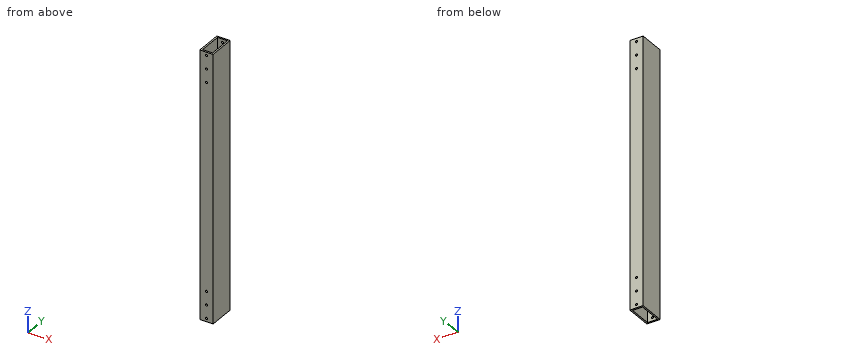
Autodesk Inventor part; units mm, degrees
ref_plane "Start Plane" through (0, 0, 0) normal (0, 0, 1) x (1, 0, 0)
ref_plane "End Plane" through (0, 0, 508) normal (0, 0, 1) x (1, 0, 0)
ref_plane "YZ Plane" through (0, 0, 0) normal (1, 0, 0) x (0, 1, 0)
ref_plane "Start Plane" through (0, 0, 0) normal (0, 0, 1) x (1, 0, 0)
ref_plane "End Plane" through (0, 0, 508) normal (0, 0, 1) x (1, 0, 0)
sketch "Sketch" plane through (0, 0, 0) normal (0, 0, 1) x (1, 0, 0)
  line L0 (-12.7, -25.4) -> (12.7, -25.4)
  line L1 (12.7, -25.4) -> (12.7, 25.4)
  line L2 (12.7, 25.4) -> (-12.7, 25.4)
  line L3 (-12.7, 25.4) -> (-12.7, -25.4)
  line L4 (-12.7, -25.4) -> (12.7, 25.4) construction
  line L5 (12.7, -25.4) -> (-12.7, 25.4) construction
  line L6 (-9.525, -22.225) -> (9.525, -22.225)
  line L7 (9.525, -22.225) -> (9.525, 22.225)
  line L8 (9.525, 22.225) -> (-9.525, 22.225)
  line L9 (-9.525, 22.225) -> (-9.525, -22.225)
  line L10 (-9.525, -22.225) -> (9.525, 22.225) construction
  line L11 (9.525, -22.225) -> (-9.525, 22.225) construction
  point P0 (0, 0)
  dimension "d0" = 25.4
  dimension "d1" = 50.8
  dimension "d2" = 3.175
  dimension "d3" = 3.175
extrude "Body" add sketch "Sketch" along normal up to surface (508 mm away) from surface at 0
sketch "Sketch6" plane through (0, 0, 0) normal (0, 0, 1) x (1, 0, 0)
  line L0 (0, 0) -> (10, 0)
ref_plane "Work Plane5" through (0, 0, 0) normal (0, -1, 0) x (1, 0, 0)
sketch "Sketch7" plane through (0, 0, 0) normal (0, -1, 0) x (1, 0, 0)
  line L0 (-2, 0) -> (12, 0)
  line L1 (-2, 508) -> (12, 508)
  dimension "d11" = 508
sketch "Sketch8" plane through (-12.7, 25.4, 508) normal (0, 1, 0) x (1, 0, 0)
  point P0 (12.7, 508)
sketch "Sketch9" plane through (-12.7, 25.4, 508) normal (0, 1, 0) x (1, 0, 0)
  line L0 (0, 508) -> (25.4, 508)
  line L1 (0, 0) -> (25.4, 0)
  point P0 (12.7, 508)
  point P1 (12.7, 501.65)
  point P2 (12.7, 476.25)
  point P3 (12.7, 450.85)
  point P4 (12.7, 6.35)
  point P5 (12.7, 31.75)
  point P6 (12.7, 57.15)
  point P7 (12.7, 0)
  dimension "d16" = 6.35
  dimension "d17" = 25.4
  dimension "d18" = 25.4
  dimension "d19" = 6.35
  dimension "d20" = 25.4
  dimension "d21" = 25.4
hole "Hole1" at (0, 25.4, 501.65) at (0, 25.4, 476.25) at (0, 25.4, 450.85) at (0, 25.4, 57.15) at (0, 25.4, 31.75) at (0, 25.4, 6.35) direction (0, -1, 0) diameter 4.3053 depth 50.8 tip angle 118
equation "\"d0\" = Width"
equation "\"d1\" = Height"
equation "\"d2\" = Thickness"
equation "\"d3\" = Thickness"
equation "\"Height\" = 50.8"
equation "\"Width\" = 25.4"
equation "\"Thickness\" = 3.175"
equation "\"BaseLength\" = 508"
equation "\"G_OFFSET_START\" = 0"
equation "\"G_OFFSET_END\" = 0"
equation "\"d7\" = BaseLength + G_OFFSET_END"
equation "\"G_L\" = d11"
properties part number "AL RECT TUBE 2 x 1 x 0.125" material "Aluminum 6061"
Check sheet for the modelled part. Datum: model origin and axes. Units: mm. Give positions to 0.01 mm unless a question says otherwise; leave off trailing zeros. Order: outer loops, then holes, each group sorted by start corner. A loop starts at its lowest first (then second) coordinate and runs counter-clockwise, first axis right, second up. Notation, with made-up numbers: M 65.25,43.25 L 79.25,43.25 A33 cw 79.25,82.25 Z; hole C -36.75,-25.75 d7. An arc over 180 degrees is marked long. Answer in a Markdown table with one row per item.
1) Cross-section at B-B, the plane z = 362. Enter the section's corners in (x, y) (3 decimals), plus the area to 3 significant figures.
Filled sheet:
| item | result |
|---|---|
| outline | M -12.7,-25.4 L 12.7,-25.4 L 12.7,25.4 L -12.7,25.4 Z; hole M -9.525,-22.225 L 9.525,-22.225 L 9.525,22.225 L -9.525,22.225 Z |
| area | 444 mm2 |
2) Thickness scan on L1, parallel to X at y = -5.5, z = 312.5 (3 decimals); L2, parallel to Y at x = 8.75, z = 316.5 (3 decimals); L3, parallel to X at y = 24.1, z = 57.15. Record the ranges inside material, lowest first. Write a range as [from, to].
Filled sheet:
| item | result |
|---|---|
| L1 | x = [-12.7, -9.525], [9.525, 12.7] |
| L2 | y = [-25.4, -22.225], [22.225, 25.4] |
| L3 | x = [-12.7, -2.15], [2.15, 12.7] |
3) Gauge pin test, flat end, axial feed: P1, Ø5, axis at x = 0, z = 6.35, coming from the +Y side. Record the tip position at first contact, or that the pin passes through.
Filled sheet:
| item | result |
|---|---|
| P1 | stops at y = 25.4 |
4) Cross-section at A-A, the plane y = -13.5. Enter the section's corners in (x, z) (3 decimals).
Filled sheet:
| item | result |
|---|---|
| outline | M -12.7,0 L -9.525,0 L -9.525,508 L -12.7,508 Z; M 9.525,0 L 12.7,0 L 12.7,508 L 9.525,508 Z |
